```python
from build123d import *

# Parameters (mm, degrees)
CROQUIS1_W              = 25
CROQUIS1_H              = 3
SALIENTE_EXTRUIR1_DEPTH = 195
CROQUIS2_R              = 4.25
CORTAR_EXTRUIR1_DEPTH   = 195
CROQUIS3_W              = 4
CROQUIS3_H              = 25
SALIENTE_EXTRUIR2_DEPTH = 195
SALIENTE_EXTRUIR3_START = 1
CROQUIS4_W              = 29
CROQUIS4_H              = 195
CROQUIS4_R              = 4.25
SALIENTE_EXTRUIR3_DEPTH = 1
CROQUIS5_W              = 149.811438776
CROQUIS5_H              = 152
CORTAR_EXTRUIR4_DEPTH   = 40
CROQUIS6_R              = 4.25
CORTAR_EXTRUIR5_DEPTH   = 40
SALIENTE_EXTRUIR4_DEPTH = 4


with BuildPart() as part:
    # Croquis1 → Saliente-Extruir1 (new body)
    with BuildSketch(Plane(origin=(0, 0, 0), x_dir=(1, 0, 0), z_dir=(0, 1, 0))):
        with Locations((12.5, -1.5)):
            Rectangle(CROQUIS1_W, CROQUIS1_H)
    extrude(amount=SALIENTE_EXTRUIR1_DEPTH)

    # Croquis2 → Cortar-Extruir1 (cut)
    with BuildSketch(Plane.XY.offset(3)):
        with Locations((18.25, 180)):
            Circle(CROQUIS2_R)
        with Locations((18.25, 97.5)):
            Circle(CROQUIS2_R)
        with Locations((18.25, 15)):
            Circle(CROQUIS2_R)
    extrude(amount=-CORTAR_EXTRUIR1_DEPTH, mode=Mode.SUBTRACT)

    # Croquis3 → Saliente-Extruir2 (add)
    with BuildSketch(Plane(origin=(0, 195, 0), x_dir=(1, 0, 0), z_dir=(0, 1, 0))):
        with Locations((-2, 9.5)):
            Rectangle(CROQUIS3_W, CROQUIS3_H)
    extrude(amount=-SALIENTE_EXTRUIR2_DEPTH)

    # Croquis4 → Saliente-Extruir3 (add)
    with BuildSketch(Plane.XY.offset(3).offset(SALIENTE_EXTRUIR3_START)):
        with Locations((10.5, 97.5)):
            Rectangle(CROQUIS4_W, CROQUIS4_H)
        with Locations((18.25, 15)):
            Circle(CROQUIS4_R, mode=Mode.SUBTRACT)
        with Locations((18.25, 97.5)):
            Circle(CROQUIS4_R, mode=Mode.SUBTRACT)
        with Locations((18.25, 180)):
            Circle(CROQUIS4_R, mode=Mode.SUBTRACT)
    extrude(amount=-SALIENTE_EXTRUIR3_DEPTH)

    # Croquis5 → Cortar-Extruir4 (cut)
    with BuildSketch(Plane.XY.offset(4)):
        with Locations((-49.905719388, 76)):
            Rectangle(CROQUIS5_W, CROQUIS5_H)
    extrude(amount=-CORTAR_EXTRUIR4_DEPTH, mode=Mode.SUBTRACT)

    # Croquis6 → Cortar-Extruir5 (cut)
    with BuildSketch(Plane.XY.offset(4)):
        with Locations((18.25, 173.5)):
            Circle(CROQUIS6_R)
    extrude(amount=-CORTAR_EXTRUIR5_DEPTH, mode=Mode.SUBTRACT)

    # Croquis7 → Saliente-Extruir4 (add)
    with BuildSketch(Plane.XY.offset(4)):
        with BuildLine():
            ThreePointArc((20.988612788, 176.75), (22.103673854, 178.207878959), (22.5, 180))
            ThreePointArc((22.5, 180), (16.457878959, 183.853673854), (15.511387212, 176.75))
            ThreePointArc((15.511387212, 176.75), (18.25, 177.75), (20.988612788, 176.75))
        make_face()
    extrude(amount=-SALIENTE_EXTRUIR4_DEPTH)


solid = part.part
```
Design review of the part built by this model. Coordinates are the model's own, in mm. A direction names the side the tool comes from. Coordinates: 2 decimals unless noted, no trailing zeros. Loops run counter-clockwise (first coordinate to the right, second up) from the corner with the lowest first, then second, coordinate; pieces in that order, holes last. Notation, with made-up numbers: (33, 4) -> (47, 4) arc R15 cw to (47, 27) -> close; hole circle Ø9 at (18.5, 81.5). An arc over 180 degrees is marked (long way). Answer as a JSON object with one key per item and string values.
Q1. Clearance check with flat-ended pins moving along their axes: pin 1 Ø4 at (x, y) = (21.5, 183) entering from -Z; pin 2 Ø11 at (x, y) = (18.25, 173.5) entering from +Z; pin 3 Ø12 at (y, z) = (170, -8) entering from +X. State where each tip first meets the part, or that it passes through.
Answer block:
{"pin 1": "stops at z = 0", "pin 2": "stops at z = 4", "pin 3": "stops at x = 0"}
Q2. Take a section at D-D on y = 165. Give the boundary of the cut face in (x, z).
Answer block:
{"outline": "(-4, -22) -> (0, -22) -> (0, 0) -> (25, 0) -> (25, 4) -> (-4, 4) -> close"}
Q3. Take a section at B-B on x = 18.25. Give the boundary of the cut face in (y, z).
Answer block:
{"outline": "(152, 0) -> (169.25, 0) -> (169.25, 4) -> (152, 4) -> close; (177.75, 0) -> (195, 0) -> (195, 4) -> (177.75, 4) -> close"}
Q4. Take a section at A-A on y = 173.5. Give the boundary of the cut face in (x, z), plus the area to 3 significant figures.
Answer block:
{"outline": "(-4, -22) -> (0, -22) -> (0, 0) -> (14, 0) -> (14, 4) -> (-4, 4) -> close; (22.5, 0) -> (25, 0) -> (25, 4) -> (22.5, 4) -> close", "area": "170 mm^2"}
Q5. Tool access review of faces 1 (the flat face through (12, 174, 0)), 2 (the flat face through (-2, 174, -22)): name each direction out of +Z, -Z, +X, -X, +Y, -Y from which nothing blocks a thin tool from reaching the whole face with its end or side.
Answer block:
{"face 1": "-Z, +X, +Y, -Y", "face 2": "-Z, +X, -X, +Y, -Y"}
Q6. To check wall thickness, follow L1, parallel to X at y = 173.5, z = 0.9; L2, parallel to Y at x = 18.25, z = 3.05; L3, parallel to X at y = 180, z = -9.25. State the ranges of each line that lie inside material, in increasing order.
Answer block:
{"L1": "x = -4 to 14, 22.5 to 25", "L2": "y = 152 to 169.25, 177.75 to 195", "L3": "x = -4 to 0"}
Q7. Take a section at C-C on z = -17.75. Give the boundary of the cut face in (x, y), plus the area to 3 significant figures.
Answer block:
{"outline": "(-4, 152) -> (0, 152) -> (0, 195) -> (-4, 195) -> close", "area": "172 mm^2"}
